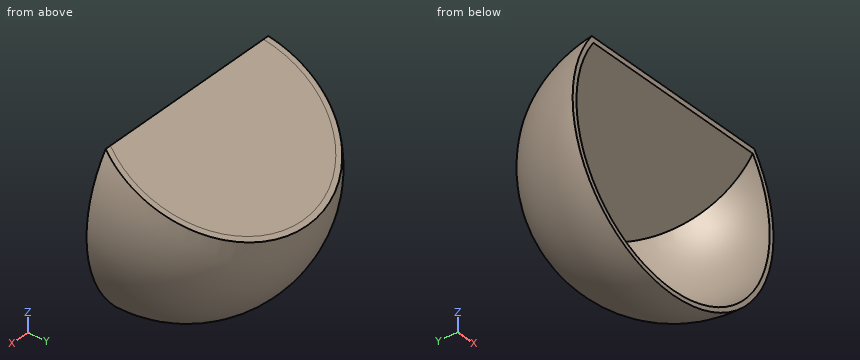
```python
from build123d import *

# Parameters (mm, degrees)
R_VOLUTION1_ANGLE            = 180
COQUE4_T                     = -4
ENL_V_MAT_EXTRU_4_DEPTH      = 215
ENL_V_MAT_EXTRU_4_DEPTH_BACK = 215
BOSS_EXTRU_2_DEPTH           = 4
ENL_V_MAT_EXTRU_5_DEPTH      = 116
ENL_V_MAT_EXTRU_5_DEPTH_BACK = 116


with BuildPart() as part:
    # Esquisse3 → Révolution1 (revolve)
    with BuildSketch(Plane(origin=(0, 0, 0), x_dir=(1, 0, 0), z_dir=(0, 1, 0))):
        with BuildLine():
            Line((-99.218538531, -45.831289244), (92.520591904, -45.831289244))
            Line((92.520591904, -45.831289244), (101.651026687, -45.831289244))
            ThreePointArc((101.651026687, -45.831289244), (-3.348973313, 59.168710756), (-108.348973313, -45.831289244))
            Line((-108.348973313, -45.831289244), (-99.218538531, -45.831289244))
        make_face()
    revolve(axis=Axis((-99.218538531, 0, 45.831289244), (1, 0, 0)), revolution_arc=R_VOLUTION1_ANGLE)

    # Coque4
    coque4_openings = [part.faces().sort_by_distance(p)[0] for p in [
        (-3.348973313, 0, 45.831289244),
    ]]
    offset(amount=COQUE4_T, openings=coque4_openings)

    # Esquisse8 → Enlèv. mat.-Extru.4 (cut, two sides: drawn at the far end of the back side and taken through both)
    with BuildSketch(Plane(origin=(60.188697083, -79.696891645, -906.524570727), x_dir=(0, 0, -1), z_dir=(1, 0, 0)).offset(-ENL_V_MAT_EXTRU_4_DEPTH_BACK)):
        Polygon((-1014, 79.696891645), (-952.35585997, 184.696891645), (-1018.029052905, 190.459065972), (-1080.678095687, 148.38135067), (-1080.678095687, 69.088233835), align=None)
    extrude(amount=ENL_V_MAT_EXTRU_4_DEPTH + ENL_V_MAT_EXTRU_4_DEPTH_BACK, mode=Mode.SUBTRACT)

    # Esquisse9 → Boss.-Extru.2 (add)
    with BuildSketch(Plane(origin=(0, 46.924060253, 79.926921264), x_dir=(1, 0, 0), z_dir=(0, 0.5062842851630452, 0.8623666404708291))):
        with BuildLine():
            Line((-88.348973313, -54.413120882), (81.651026687, -54.413120882))
            ThreePointArc((81.651026687, -54.413120882), (-3.348973313, 67.344835737), (-88.348973313, -54.413120882))
        make_face()
    extrude(amount=-BOSS_EXTRU_2_DEPTH)

    # Esquisse12 → Enlèv. mat.-Extru.5 (cut, two sides: drawn at the far end of the back side and taken through both)
    with BuildSketch(Plane(origin=(0, 0, 0), x_dir=(0, 0, -1), z_dir=(1, 0, 0)).offset(-ENL_V_MAT_EXTRU_5_DEPTH_BACK)):
        Polygon((-107.475429273, 0), (-102.191678846, 0), (-103.675762979, -3.693901999), align=None)
    extrude(amount=ENL_V_MAT_EXTRU_5_DEPTH + ENL_V_MAT_EXTRU_5_DEPTH_BACK, mode=Mode.SUBTRACT)


solid = part.part
```
Could you check a few things on this model? Use its own coordinates, in mm. Give positions to 0.01 mm unless a question says otherwise; leave off trailing zeros. Order: outer loops, then holes, each group sorted by start corner. A loop starts at its lowest first (then second) coordinate and runs counter-clockwise, first axis right, second up.
Q1. Suppose I cut it at C-C, the plane z = 82.5. Write out the boundary of the cut face in (x, y), and give its area (3 significant figures).
Q2. Suppose I cut it at A-A, the plane x = -10.5. Write out the boundary of the cut face in (y, z).
Q3. Suppose I cut it at D-D, the plane y = 59.5. Write out the boundary of the cut face in (x, z), and give its area (3 significant figures).
Q4. I'm going to push flat-ended pins straight in: P1, Ø12, axis at x = 52.5, y = 78, coming from the +Z side; P2, Ø6, axis at x = 45.5, z = 34.5, coming from the +Y side; P3, Ø10, axis at y = 81.5, z = -12, coming from the -X side. Where does each tip first touch, or does it pass through?
Q5. If I drill on line 1 along Z through (x, y) = (-58.5, 14); line 2 along X through (y, z) = (80, 19.5); line 3 along X through (y, z) = (64.5, 32), over which ranges is the centre line in solid material (lowest first)?
Q6. Suppose I cut it at B-B, the plane y = 47.5. Write out the boundary of the cut face in (x, z).
Solution:
1. outline: (-101.74, 0) - (-97.46, 0) arc R94.11 cw to (-90.85, 34.64) - (84.15, 34.64) arc R94.11 cw to (90.76, 0) - (95.04, 0) arc R98.39 ccw to (85.37, 42.54) - (-92.07, 42.54) arc R98.39 ccw to start
1. area: 1,730 mm2
2. outline: (0, -58.92) arc R104.76 ccw to (104.76, 45.97) - (0, 107.48) - (0, 102.84) - (100.72, 43.7) arc R100.75 cw to (0, -54.92) - close
3. outline: (-85.64, 72.54) arc R86.51 ccw (long way) to (78.94, 72.54) - close; hole (-81.92, 67.91) arc R81.61 ccw (long way) to (75.22, 67.91) - close
3. area: 2,280 mm2
4. P1: stops at z = 65.21
4. P2: stops at y = 93.82
4. P3: stops at x = -48.21
5. line 1: z = -42.41 to -37.62, 94.62 to 99.26
5. line 2: x = -66.05 to -59.1, 52.4 to 59.35
5. line 3: x = -85.04 to -79.83, 73.13 to 78.34
6. outline: (-90.69, 79.59) arc R93.64 ccw (long way) to (84, 79.59) - close; hole (-87.59, 74.95) arc R89.13 ccw (long way) to (80.89, 74.95) - close
